from build123d import *

# Parameters (mm, degrees)
SKETCH1_W           = 26.998079416
SKETCH1_H           = 26.998079416
BOSS_EXTRUDE1_DEPTH = 6.35


with BuildPart() as part:
    # Sketch1 → Boss-Extrude1 (new body)
    with BuildSketch(Plane(origin=(0, 0, 0), x_dir=(1, 0, 0), z_dir=(0, 1, 0))):
        Rectangle(SKETCH1_W, SKETCH1_H)
        Polygon((6.19125, 3.574519854), (0, 7.149039708), (-6.19125, 3.574519854), (-6.19125, -3.574519854), (0, -7.149039708), (6.19125, -3.574519854), align=None, mode=Mode.SUBTRACT)
    extrude(amount=-BOSS_EXTRUDE1_DEPTH)


solid = part.part
Check sheet for the modelled part. Datum: model origin and axes. Units: mm. A direction names the side the tool comes from. Round coordinates to 2 decimals unless told otherwise and drop trailing zeros. Loops run counter-clockwise (first coordinate to the right, second up) from the corner with the lowest first, then second, coordinate; pieces in that order, holes last. Notation, with made-up numbers: M 59.25,-31.75 L 80.25,-31.75 A20 ccw 80.25,-1.75 Z; hole C -7,3 d11. An arc over 180 degrees is marked long. One line per item, written item: value.
(1) Access from +Z, -Z, +X, -X, +Y, -Y to the whole of each face (thin tool, end or side, straight path). Record for faces 1 (the face through (3.139, -3.131, -5.337)), 2 (the face through (0, -3, 13.499)).
Computed values:
face 1: +Y, -Y
face 2: +Z, +X, -X, +Y, -Y
(2) Sectioned sample at B-B, the plane y = -0.5. Record the cut outline in (x, z), then the cut area to 3 significant figures.
Computed values:
outline: M -13.5,-13.5 L 13.5,-13.5 L 13.5,13.5 L -13.5,13.5 Z; hole M -6.19,-3.57 L 0,-7.15 L 6.19,-3.57 L 6.19,3.57 L 0,7.15 L -6.19,3.57 Z
area: 596 mm^2
(3) Sectioned sample at C-C, the plane x = 3.75. Record the cut outline in (y, z), then the cut area to 3 significant figures.
Computed values:
outline: M -6.35,-13.5 L 0,-13.5 L 0,-4.98 L -6.35,-4.98 Z; M -6.35,4.98 L 0,4.98 L 0,13.5 L -6.35,13.5 Z
area: 108 mm^2
(4) Thickness scan on line 1 (Z direction, x = -4, y = -4); line 2 (Z direction, x = -5, y = -3.5); line 3 (X direction, y = -3.75, z = 1). Record the ranges inside material, lowest first.
Computed values:
line 1: z = -13.5 to -4.84, 4.84 to 13.5
line 2: z = -13.5 to -4.26, 4.26 to 13.5
line 3: x = -13.5 to -6.19, 6.19 to 13.5
(5) Sectioned sample at A-A, the plane z = -3. Record the cut outline in (x, y), then the cut area to 3 significant figures.
Computed values:
outline: M -13.5,-6.35 L -6.19,-6.35 L -6.19,0 L -13.5,0 Z; M 6.19,-6.35 L 13.5,-6.35 L 13.5,0 L 6.19,0 Z
area: 92.8 mm^2
